Answer from the drawing. Dimensions are ordinates in mm from the lowest x, y and z of the part. A direction names the side the tool comes from. Round coordinates to 2 decimals unless told otherwise and drop trailing zeros. Loops run counter-clockwise (first coordinate to the right, second up) from the corner with the lowest first, then second, coordinate; pieces in that order, holes last. Notation, with made-up numbers: M 62.25,19 L 75.25,19 A19 ccw 75.25,51 Z; hole C -7,86 d2. An arc over 180 degrees is marked long. Answer as a JSON object with one key per item and string values.
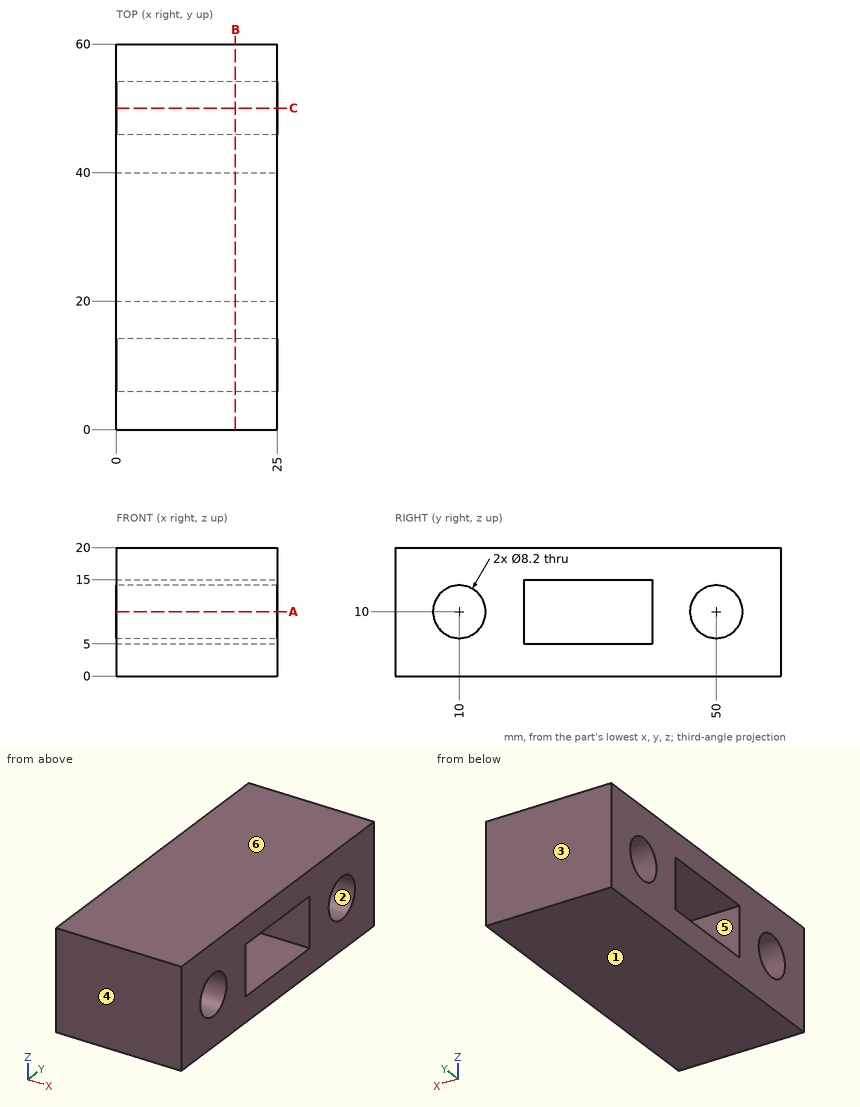
Item 1: Which of the six approach directions +Z, -Z, +X, -X, +Y, -Y give full straight-line access (tool end or side, diameter ignored) to the marked faces 5 and 6?
Values follow:
{"face 5": "+X, -X", "face 6": "+Z, +X, -X, +Y, -Y"}
Item 2: Determine the mould class of the marked faces 1, 2, 3 and 4 for opening direction Y: released by +Y, released by -Y, zero draft, split by the parting line, or undercut.
Values follow:
{"face 1": "zero draft", "face 2": "undercut", "face 3": "released by +Y", "face 4": "released by -Y"}
Item 3: A flat-ended cylindrical pin translates along its axis: P1, Ø5, axis at y = 50, z = 10, coming from the +X side. Find the tip coordinate at first contact, or state that the pin passes through.
Values follow:
{"P1": "through"}
Item 4: The part is cut by section B-B (x = 18.5). Give the vertices of the cut face in (y, z), then the cut area to 3 significant figures.
Values follow:
{"outline": "M 0,0 L 60,0 L 60,20 L 0,20 Z; hole C 10,10 d8.2; hole M 20,5 L 40,5 L 40,15 L 20,15 Z; hole C 50,10 d8.2", "area": "894 mm^2"}
Item 5: The part is cut by section A-A (z = 10). Give the vertices of the cut face in (x, y).
Values follow:
{"outline": "M 0,0 L 25,0 L 25,5.9 L 0,5.9 Z; M 0,14.1 L 25,14.1 L 25,20 L 0,20 Z; M 0,40 L 25,40 L 25,45.9 L 0,45.9 Z; M 0,54.1 L 25,54.1 L 25,60 L 0,60 Z"}
Item 6: The part is cut by section C-C (y = 50). Give the vertices of the cut face in (x, z).
Values follow:
{"outline": "M 0,0 L 25,0 L 25,5.9 L 0,5.9 Z; M 0,14.1 L 25,14.1 L 25,20 L 0,20 Z"}
Item 7: Straight lines are drawn through the part: line 1 (Y direction, x = 11.5, z = 10); line 2 (Z direction, x = 17.5, y = 21); line 3 (Y direction, x = 12.5, z = 12.25). For each, find the intervals that lie inside material, in ascending order.
Values follow:
{"line 1": "0 to 5.9, 14.1 to 20, 40 to 45.9, 54.1 to 60", "line 2": "0 to 5, 15 to 20", "line 3": "0 to 6.57, 13.43 to 20, 40 to 46.57, 53.43 to 60"}
